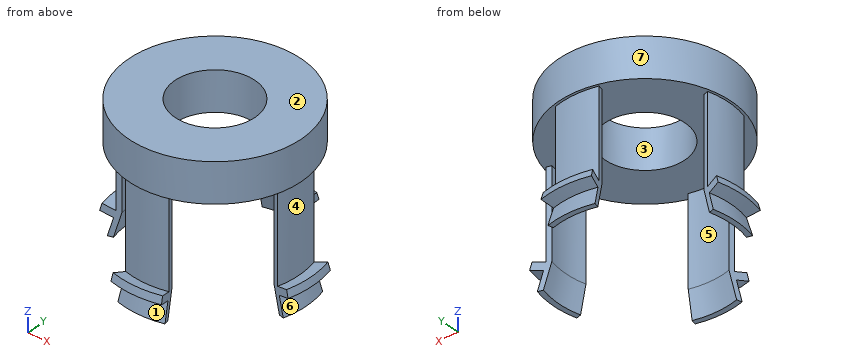
```python
from build123d import *

# Parameters (mm, degrees)
F2_R     = 17.5
F2_R_2   = 8.1
F3_DEPTH = 8
F5_DEPTH = 23


with BuildPart() as f1:
    # F0 (on Front) → F1 (revolve)
    with BuildSketch(Plane.XZ):
        Polygon((-16, 5), (-16, 23), (-17, 23), (-17, 5.142857), (-17.42, 3.702857), (-18.5, 0), (-17.458333, 0), align=None)
        Polygon((-17.42, 3.702857), (-17, 5.142857), (-19.4, 5.842857), (-19.82, 4.402857), align=None)
    revolve(axis=Axis((0, 0, 7.142946), (0, 0, 1)))

    # F2 (on face) → F3 (join)
    with BuildSketch(Plane.XY.offset(23)):
        Circle(F2_R)
        Circle(F2_R_2, mode=Mode.SUBTRACT)
    extrude(amount=F3_DEPTH)

    # F4 (on Top) → F5 (cut, through all)
    with BuildSketch(Plane.XY):
        with BuildLine():
            Line((0, 0), (-21.733331, -5.823429))
            ThreePointArc((-21.733331, -5.823429), (-15.909903, -15.909903), (-5.823429, -21.733331))
            Line((-5.823429, -21.733331), (0, 0))
        make_face()
        with BuildLine():
            Line((-21.733331, 5.823429), (0, 0))
            Line((0, 0), (-5.823429, 21.733331))
            ThreePointArc((-5.823429, 21.733331), (-15.909903, 15.909903), (-21.733331, 5.823429))
        make_face()
        with BuildLine():
            Line((5.823429, 21.733331), (0, 0))
            Line((0, 0), (21.733331, 5.823429))
            ThreePointArc((21.733331, 5.823429), (15.909903, 15.909903), (5.823429, 21.733331))
        make_face()
        with BuildLine():
            Line((21.733331, -5.823429), (0, 0))
            Line((0, 0), (5.823429, -21.733331))
            ThreePointArc((5.823429, -21.733331), (15.909903, -15.909903), (21.733331, -5.823429))
        make_face()
    extrude(amount=F5_DEPTH, mode=Mode.SUBTRACT)


solid = f1.part
```
Work out the finished part from the listing and answer in its coordinate system (mm). Face numbers are marked on the shaded views. A direction names the side the tool comes from. Round coordinates to 2 decimals unless told otherwise and drop trailing zeros. Order: outer loops, then holes, each group sorted by start corner. A loop starts at its lowest first (then second) coordinate and runs counter-clockwise, first axis right, second up.
Q1. Find the intervals of material crossed by line 1 along Y through (x, z) = (0, 25); line 2 along X through (y, z) = (2, 13.5); line 3 along Y through (x, z) = (-4.5, 29.5), in increasing order.
Solution:
line 1: y = -17.5 to -8.1, 8.1 to 17.5
line 2: x = -16.88 to -15.87, 15.87 to 16.88
line 3: y = -16.91 to -6.73, 6.73 to 16.91
Q2. A cutting plane is placed at A-A, the plane z = 17. Determine the outline of the cut face in (x, y), then the cut area to 3 significant figures.
Solution:
outline: (-16.42, -4.4) - (-15.45, -4.14) arc R16 cw to (-15.45, 4.14) - (-16.42, 4.4) arc R17 ccw to start; (-4.4, -16.42) arc R17 ccw to (4.4, -16.42) - (4.14, -15.45) arc R16 cw to (-4.14, -15.45) - close; (-4.4, 16.42) - (-4.14, 15.45) arc R16 cw to (4.14, 15.45) - (4.4, 16.42) arc R17 ccw to start; (15.45, -4.14) - (16.42, -4.4) arc R17 ccw to (16.42, 4.4) - (15.45, 4.14) arc R16 cw to start
area: 34.6 mm2
Q3. A cutting plane is placed at B-B, the plane x = 0. Determine the outline of the cut face in (y, z).
Solution:
outline: (-19.82, 4.4) - (-17.42, 3.7) - (-18.5, 0) - (-17.46, 0) - (-16, 5) - (-16, 23) - (-8.1, 23) - (-8.1, 31) - (-17.5, 31) - (-17.5, 23) - (-17, 23) - (-17, 5.14) - (-19.4, 5.84) - close; (8.1, 23) - (16, 23) - (16, 5) - (17.46, 0) - (18.5, 0) - (17.42, 3.7) - (19.82, 4.4) - (19.4, 5.84) - (17, 5.14) - (17, 23) - (17.5, 23) - (17.5, 31) - (8.1, 31) - close
Q4. A cutting plane is placed at D-D, the plane z = 26. Determine the outline of the cut face in (x, y), then the cut area to 3 significant figures.
Solution:
outline: circle Ø35 at (0, 0); hole circle Ø16.2 at (0, 0)
area: 756 mm2
Q5. Given pin 1 Ø6 at (x, z) = (3.5, 11.5) entering from -Y; pin 2 Ø10 at (x, z) = (1, 24.5) entering from +Y; pin 3 Ø3 at (x, y) = (14, 3) entering from -Z, each flat-ended and moving along its own axis, determine where each tip first touches the part or whether it passes through.
Solution:
pin 1: stops at y = -16.99
pin 2: stops at y = 17.5
pin 3: stops at z = 23
Q6. The mould has two halves that part along Z. Classify the marked faces 1, 2, 3 and 4: pulls with the +Z half, pulls with the -Z half, needs draft (parallel to the pull), parting line crosses it, or undercut.
Solution:
face 1: undercut
face 2: pulls with the +Z half
face 3: needs draft
face 4: undercut
Q7. A tool of negligible diameter and unlimited length cuts with its end or side. For the marked faces 5, 6 and 7, from which of +Z, -Z, +X, -X, +Y, -Y can it reach the whole face along a straight path? Write none if from no direction.
Solution:
face 5: -Z
face 6: +X
face 7: +Z
